Design review of the part built by this model. Coordinates are the model's own, in mm. A direction names the side the tool comes from. Give positions to 0.01 mm unless a question says otherwise; leave off trailing zeros. Loops run counter-clockwise (first coordinate to the right, second up) from the corner with the lowest first, then second, coordinate; pieces in that order, holes last. Notation, with made-up numbers: (21, -31.5) -> (46, -31.5) arc R30 ccw to (46, -3.5) -> close; hole circle Ø6 at (16.5, 88). An arc over 180 degrees is marked (long way). Answer as CSV lines item,"result".
from build123d import *

# Parameters (mm, degrees)
BOSS_EXTRUDE1_DEPTH = 1.5
CUT_EXTRUDE1_DEPTH  = 69.98434605
CHAMFER1_SIZE2      = 1.091910703
CHAMFER1_SIZE       = 3


with BuildPart() as part:
    # Sketch1 → Boss-Extrude1 (new, symmetric)
    with BuildSketch(Plane.XY):
        Polygon((-45, 0), (45, 0), (35.5, 52.2), (-35.5, 52.2), align=None)
    extrude(amount=BOSS_EXTRUDE1_DEPTH, both=True)

    # Sketch2 → Cut-Extrude1 (cut, through all)
    with BuildSketch(Plane.XY.offset(1.5)):
        with BuildLine():
            Line((-17.5, 29.2), (-17.5, 19.2))
            ThreePointArc((-17.5, 19.2), (-25, 11.7), (-32.5, 19.2))
            Line((-32.5, 19.2), (-32.5, 29.2))
            ThreePointArc((-32.5, 29.2), (-25, 36.7), (-17.5, 29.2))
        make_face()
        with BuildLine():
            Line((17.5, 29.2), (17.5, 19.2))
            ThreePointArc((17.5, 19.2), (25, 11.7), (32.5, 19.2))
            Line((32.5, 19.2), (32.5, 29.2))
            ThreePointArc((32.5, 29.2), (25, 36.7), (17.5, 29.2))
        make_face()
    extrude(amount=-CUT_EXTRUDE1_DEPTH, mode=Mode.SUBTRACT)

    # Chamfer1
    chamfer1_edges = [part.edges().sort_by_distance(p)[0] for p in [
        (0, 0, -1.5),
    ]]
    chamfer1_side = [part.faces().sort_by_distance(p)[0] for p in [
        (0, 0, -1.478161786),
    ]]
    chamfer(chamfer1_edges, length=CHAMFER1_SIZE - 0.0001, length2=CHAMFER1_SIZE2 - 0.0001, reference=chamfer1_side[0])  # a hair under: the kernel refuses the full size


solid = part.part
Q1. For faces 5 (the flat face through (17.5, 24, 0)), 6 (the flat face through (-0.63, 0.554, -0.021)), list the 3-axis set-ups (+Z, -Z, +X, -X, +Y, -Y) from which the entire face can be reached by the end or side of a thin tool; tool diameter is ignored.
Filled sheet:
face 5,"+Z, -Z"
face 6,"-Z, +X, -X, -Y"
Q2. We need section B-B, the plane y = 24. State the section outline as (x, z) points, and give its area (3 significant figures).
Filled sheet:
outline,"(-40.63, -1.5) -> (-32.5, -1.5) -> (-32.5, 1.5) -> (-40.63, 1.5) -> close; (-17.5, -1.5) -> (17.5, -1.5) -> (17.5, 1.5) -> (-17.5, 1.5) -> close; (32.5, -1.5) -> (40.63, -1.5) -> (40.63, 1.5) -> (32.5, 1.5) -> close"
area,"154 mm^2"
Q3. The part is to be moulded in two halves that separate along X. For faces 1 (the flat face through (0, 52.2, 0)), 2 (the flat face through (40.316, 25.735, 0.021)), 3 (the cylindrical face through (24.84, 11.7, 0.02)), 4 (the flat face through (-40.184, 26.465, 0.021)), say which applies: pulls with the +X half, pulls with the -X half, needs draft (parallel to the pull), parting line crosses it, or undercut.
Filled sheet:
face 1,"needs draft"
face 2,"pulls with the +X half"
face 3,"undercut"
face 4,"pulls with the -X half"
Q4. To check wall thickness, follow probe 1 along X at (y, z) = (21, 0.95); probe 2 along X at (y, z) = (29, 0.45); probe 3 along Y at (x, z) = (26, -0.8). State the ranges of each line that lie inside material, in increasing order. Write a range as from..to.
Filled sheet:
probe 1,"x = -41.18..-32.5, -17.5..17.5, 32.5..41.18"
probe 2,"x = -39.72..-32.5, -17.5..17.5, 32.5..39.72"
probe 3,"y = 0.84..11.77, 36.63..52.2"
Q5. Clearance check with a flat-ended pin moving along its axis: pin 1 Ø0.9 at (y, z) = (24.5, 0.5) entering from +X. State where the tip first meets the part, or that it passes through.
Filled sheet:
pin 1,"stops at x = 40.62"
Q6. We need section D-D, the plane y = 38. State the section outline as (x, z) points.
Filled sheet:
outline,"(-38.08, -1.5) -> (38.08, -1.5) -> (38.08, 1.5) -> (-38.08, 1.5) -> close"
Q7. We need section C-C, the plane z = -0.1. State the section outline as (x, y) points.
Filled sheet:
outline,"(-44.89, 0.58) -> (44.89, 0.58) -> (35.5, 52.2) -> (-35.5, 52.2) -> close; hole (-32.5, 19.2) arc R7.5 ccw to (-17.5, 19.2) -> (-17.5, 29.2) arc R7.5 ccw to (-32.5, 29.2) -> close; hole (17.5, 19.2) arc R7.5 ccw to (32.5, 19.2) -> (32.5, 29.2) arc R7.5 ccw to (17.5, 29.2) -> close"
